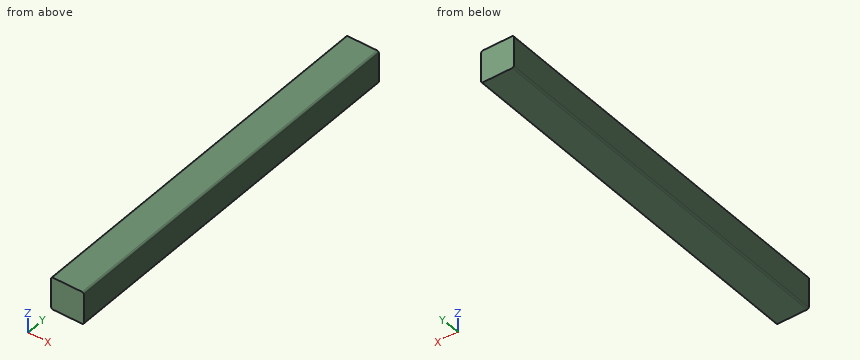
```python
from build123d import *

# Parameters (mm, degrees)
F1_DEPTH = 1155
F4_DEPTH = 20
F7_DEPTH = 10


with BuildPart() as f1:
    # F0 (on Front) → F1 (new body)
    with BuildSketch(Plane.XZ):
        with BuildLine():
            ThreePointArc((50, 45), (48.5355339059, 48.5355339059), (45, 50))
            Line((45, 50), (-45, 50))
            ThreePointArc((-45, 50), (-48.5355339059, 48.5355339059), (-50, 45))
            Line((-50, 45), (-50, -45))
            ThreePointArc((-50, -45), (-48.5355339059, -48.5355339059), (-45, -50))
            Line((-45, -50), (45, -50))
            ThreePointArc((45, -50), (48.5355339059, -48.5355339059), (50, -45))
            Line((50, -45), (50, 45))
        make_face()
        with BuildLine():
            ThreePointArc((-47, 45), (-46.4142135624, 46.4142135624), (-45, 47))
            Line((-45, 47), (45, 47))
            ThreePointArc((45, 47), (46.4142135624, 46.4142135624), (47, 45))
            Line((47, 45), (47, -45))
            ThreePointArc((47, -45), (46.4142135624, -46.4142135624), (45, -47))
            Line((45, -47), (-45, -47))
            ThreePointArc((-45, -47), (-46.4142135624, -46.4142135624), (-47, -45))
            Line((-47, -45), (-47, 45))
        make_face(mode=Mode.SUBTRACT)
    extrude(amount=-F1_DEPTH)

    # F3 (on offset) → F4 (join)
    with BuildSketch(Plane.XZ.offset(10)):
        with BuildLine():
            Line((45, 50), (-45, 50))
            ThreePointArc((-45, 50), (-48.5355339059, 48.5355339059), (-50, 45))
            Line((-50, 45), (-50, -45))
            ThreePointArc((-50, -45), (-48.5355339059, -48.5355339059), (-45, -50))
            Line((-45, -50), (45, -50))
            ThreePointArc((45, -50), (48.5355339059, -48.5355339059), (50, -45))
            Line((50, -45), (50, 45))
            ThreePointArc((50, 45), (48.5355339059, 48.5355339059), (45, 50))
        make_face()
    extrude(amount=-F4_DEPTH)

    # F6 (on offset) → F7 (join)
    with BuildSketch(Plane(origin=(0, 1165, 0), x_dir=(-1, 0, 0), z_dir=(0, 1, 0))):
        with BuildLine():
            Line((45, 50), (-45, 50))
            ThreePointArc((-45, 50), (-48.5355339059, 48.5355339059), (-50, 45))
            Line((-50, 45), (-50, -45))
            ThreePointArc((-50, -45), (-48.5355339059, -48.5355339059), (-45, -50))
            Line((-45, -50), (45, -50))
            ThreePointArc((45, -50), (48.5355339059, -48.5355339059), (50, -45))
            Line((50, -45), (50, 45))
            ThreePointArc((50, 45), (48.5355339059, 48.5355339059), (45, 50))
        make_face()
    extrude(amount=-F7_DEPTH)


solid = f1.part
```
Input: part model. Units: mm. Frame: model coordinates. Coordinates: 2 decimals unless noted, no trailing zeros. Loops run counter-clockwise (first coordinate to the right, second up) from the corner with the lowest first, then second, coordinate; pieces in that order, holes last. Notation, with made-up numbers: M 75,21.5 L 120,21.5 A18 cw 120,49.5 Z; hole C 48.25,-3 d5. An arc over 180 degrees is marked long. Answer in a Markdown table with one row per item.
1. Section B-B, the plane y = 105.5. Output: boundary loops of the cut face in (x, z).
Response:
| item | result |
|---|---|
| outline | M -50,-45 A5 ccw -45,-50 L 45,-50 A5 ccw 50,-45 L 50,45 A5 ccw 45,50 L -45,50 A5 ccw -50,45 Z; hole M -47,-45 A2 ccw -45,-47 L 45,-47 A2 ccw 47,-45 L 47,45 A2 ccw 45,47 L -45,47 A2 ccw -47,45 Z |
2. Material intervals for line 1 (Z direction, x = 40, y = 749.5); line 2 (Y direction, x = -31, z = 42.5), sorted ascending.
Response:
| item | result |
|---|---|
| line 1 | z = -50 to -47, 47 to 50 |
| line 2 | y = -10 to 10, 1155 to 1165 |
3. Section C-C, the plane x = 31.5. Output: boundary loops of the cut face in (y, z), then the cut area to 3 significant figures.
Response:
| item | result |
|---|---|
| outline | M -10,-50 L 1165,-50 L 1165,50 L -10,50 Z; hole M 10,-47 L 1155,-47 L 1155,47 L 10,47 Z |
| area | 9,870 mm2 |
4. Section A-A, the plane z = 31. Output: boundary loops of the cut face in (x, y), then the cut area to 3 significant figures.
Response:
| item | result |
|---|---|
| outline | M -50,-10 L 50,-10 L 50,1165 L -50,1165 Z; hole M -47,10 L 47,10 L 47,1155 L -47,1155 Z |
| area | 9,870 mm2 |
